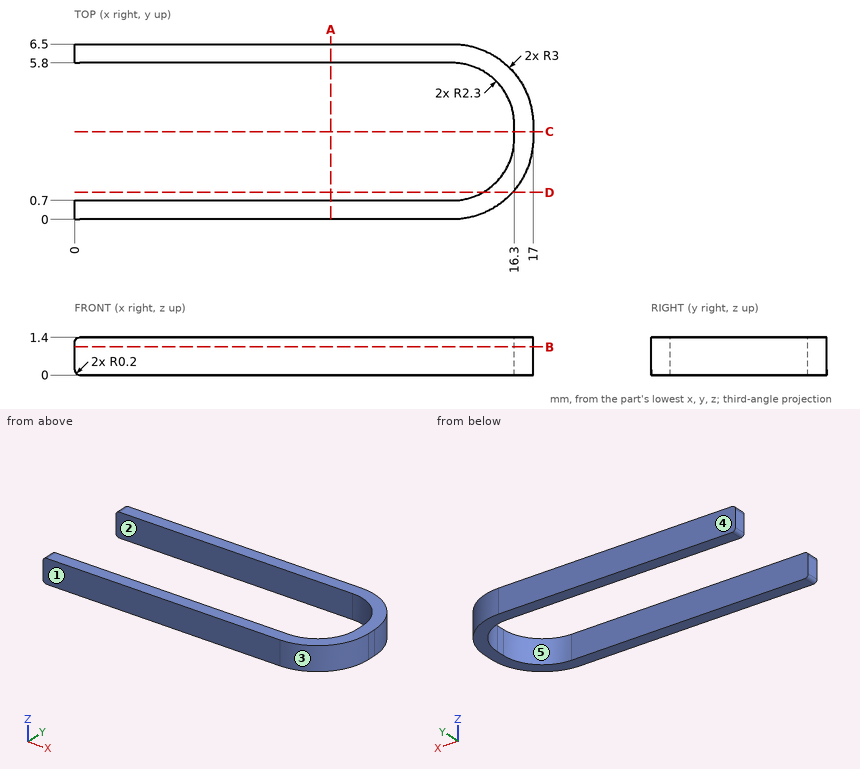
Verification items for this drawing (mm, ordinates from the low corner). A direction names the side the tool comes from. Coordinates: 2 decimals unless noted, no trailing zeros. Loops run counter-clockwise (first coordinate to the right, second up) from the corner with the lowest first, then second, coordinate; pieces in that order, holes last. Notation, with made-up numbers: (-12, -25.5) -> (40, -25.5) arc R25 ccw to (40, 0.5) -> close; hole circle Ø4 at (-24.75, 78). An arc over 180 degrees is marked (long way). Answer in a Markdown table with one row per item. Add a question column.
1. Section check D-D, the plane y = 1. Enter the section's corners in (x, z).
2. Draft check along Y on the marked faces 3, 4 and 5. Enter one of: +Y half, -Y half, draft (parallel to the pull), parting line (faces both ways), or undercut.
3. Section check A-A, the plane x = 9.5. Enter the section's corners in (y, z), then the cut area to 3 significant figures.
4. Section check C-C, the plane y = 3.25. Enter the section's corners in (x, z), then the cut area to 3 significant figures.
5. Material ranges on probe 1 along Y at (x, z) = (4, 0.35); probe 2 along X at (y, z) = (3, 0.3); probe 3 along Y at (x, z) = (14.5, 1.15) (3 decimals), recorded low to high. Write a range as [from, to].
6. Depth check by flat-ended pin: P1, Ø1, axis at x = 13, y = 1.5, coming from the -Z side. Enter the tip coordinate at first touch or a pass-through.
7. Section check B-B, the plane z = 1.05. Enter the section's corners in (x, y).
8. Access from +Z, -Z, +X, -X, +Y, -Y to the whole of each face (thin tool, end or side, straight path). Record for the marked faces 1 and 2.
Derived:
| question | item | result |
|---|---|---|
| 1 | outline | (15.14, 0) -> (16.24, 0) -> (16.24, 1.4) -> (15.14, 1.4) -> close |
| 2 | face 3 | -Y half |
| 2 | face 4 | +Y half |
| 2 | face 5 | undercut |
| 3 | outline | (0, 0) -> (0.7, 0) -> (0.7, 1.4) -> (0, 1.4) -> close; (5.8, 0) -> (6.5, 0) -> (6.5, 1.4) -> (5.8, 1.4) -> close |
| 3 | area | 1.96 mm² |
| 4 | outline | (16.3, 0) -> (17, 0) -> (17, 1.4) -> (16.3, 1.4) -> close |
| 4 | area | 0.980 mm² |
| 5 | probe 1 | y = [0, 0.7], [5.8, 6.5] |
| 5 | probe 2 | x = [16.3, 17] |
| 5 | probe 3 | y = [0.042, 0.755], [5.745, 6.458] |
| 6 | P1 | passes through |
| 7 | outline | (0, 0) -> (14, 0) arc R3 ccw to (17, 3) -> (17, 3.5) arc R3 ccw to (14, 6.5) -> (0, 6.5) -> (0, 5.8) -> (14, 5.8) arc R2.3 cw to (16.3, 3.5) -> (16.3, 3) arc R2.3 cw to (14, 0.7) -> (0, 0.7) -> close |
| 8 | face 1 | +Z, -Z, +X, -X, -Y |
| 8 | face 2 | +Z, -Z, -X |
